The model under review builds one solid part; all positions refer to its coordinate system, in mm. A direction names the side the tool comes from. Round coordinates to 2 decimals unless told otherwise and drop trailing zeros. Order: outer loops, then holes, each group sorted by start corner. A loop starts at its lowest first (then second) coordinate and runs counter-clockwise, first axis right, second up. Notation, with made-up numbers: M 77.5,88 L 128.5,88 A23 cw 128.5,115 Z; hole C 43,7 d9. An arc over 180 degrees is marked long. Answer as a JSON object with one key per item and string values. Group by question number.
1. Add section A-A on y = -9. State the section outline as (x, z) points.
2. Mouldability with a two-part tool opening along Y and no side actions: class faces 4 (the face through (-44.44, -49.53, 67.02)), 5 (the face through (3, -17, 29.674)), 6 (the face through (2, 12.931, 37)), 7 (the face through (-25, -52.069, 37)) as released by +Y, released by -Y, zero draft, split by the parting line, or undercut.
3. Machinability: for faces 1 (the face through (3, -17, 43.524)), 2 (the face through (2, -34, 75)), 3 (the face through (-27, -47.069, 37)), which of the approach directions +Z, -Z, +X, -X, +Y, -Y give a long, thin tool a straight path to every point of the face, cutting with its end or side? Answer none if there is none.
4. Clearance check with flat-ended pins moving along their axes: P1, Ø3, axis at x = -17, z = 61, coming from the +Y side; P2, Ø2.5, axis at y = -2.46, z = 36.6, coming from the -X side. State where each tip first meets the part, or that it passes through.
5. To check wall thickness, follow probe 1 along Y at (x, z) = (-36.5, 72.5); probe 2 along X at (y, z) = (-33.5, 5). State the ranges of each line that lie inside material, in increasing order. Write a range as [from, to].
6. Add section C-C on z = 67. State the section outline as (x, y) points.
7. Add section B-B on z = 31. State the section outline as (x, y) points.
8. Add section D-D on x = -19.5. State the section outline as (y, z) points, and give its area (3 significant figures).
Autodesk Inventor part; units mm, degrees
ref_plane "YZ Plane" through (0, 0, 0) normal (1, 0, 0) x (0, 1, 0)
ref_plane "XZ Plane" through (0, 0, 0) normal (0, 1, 0) x (-1, 0, 0)
ref_plane "XY Plane" through (0, 0, 0) normal (0, 0, 1) x (1, 0, 0)
sketch "Sketch1" plane through (0, 0, 0) normal (0, 0, 1) x (1, 0, 0)
  point P0 (0, 0)
sketch "Sketch2" plane through (0, 0, 0) normal (0, 0, 1) x (1, 0, 0)
  line L0 (0, 12.9308) -> (5, 12.9308)
  line L1 (5, 12.9308) -> (5, -47.0692)
  line L2 (0, -47.0692) -> (0, 12.9308)
  line L3 (0, -47.0692) -> (-55, -47.0692)
  line L4 (-55, -47.0692) -> (-55, -52.0692)
  line L5 (-55, -52.0692) -> (5, -52.0692)
  line L6 (5, -52.0692) -> (5, -47.0692)
  point P0 (0, 0)
extrude "Extrusion1" add sketch "Sketch2" along normal blind 75
sketch "Sketch3" plane through (-55, -47.0692, 0) normal (0, 1, 0) x (1, 0, 0)
  circle A0 centre (8.2492, -7.6821) radius 2.5
  circle A1 centre (8.2492, -66.0616) radius 2.5
  point P0 (55, 0)
  dimension "d6" = 5
  dimension "d7" = 5
extrude "Extrusion2" cut sketch "Sketch3" against normal blind 75
sketch "Sketch4" plane through (5, -52.0692, 0) normal (1, 0, 0) x (0, 0, -1)
  line L0 (-43.5238, 46.3128) -> (-29.6738, 46.3128)
  line L1 (-29.6738, 46.3128) -> (-29.6738, 23.4735)
  line L2 (-29.6738, 23.4735) -> (-43.5238, 23.4735)
  line L3 (-43.5238, 23.4735) -> (-43.5238, 46.3128)
  point P0 (0, 52.0692)
extrude "Extrusion3" cut sketch "Sketch4" against normal blind 75
sketch "Sketch5" plane through (5, -52.0692, 0) normal (1, 0, 0) x (0, 0, -1)
  line L0 (-43.5238, 46.3128) -> (-43.5238, 23.4735)
  line L1 (-43.5238, 46.3128) -> (-29.6738, 46.3128)
  line L2 (-43.5238, 46.3128) -> (-29.6738, 46.3128)
  line L3 (-43.5238, 46.3128) -> (-36.5988, 46.3128)
  circle A0 centre (-36.5988, 49.6128) radius 1
  circle A1 centre (-36.5988, 20.1735) radius 1
  point P0 (0, 52.0692)
extrude "Extrusion4" cut sketch "Sketch5" against normal blind 75
Recorded:
{
 "1": {"outline": "M 0,0 L 5,0 L 5,29.67 L 0,29.67 Z; M 0,43.52 L 5,43.52 L 5,75 L 0,75 Z"},
 "2": {"face 4": "zero draft", "face 5": "undercut", "face 6": "released by +Y", "face 7": "released by -Y"},
 "3": {"face 1": "+X, -X", "face 2": "+Z, +X, -X, +Y, -Y", "face 3": "+Z, -Z, -X, +Y"},
 "4": {"P1": "stops at y = -47.07", "P2": "stops at x = 0"},
 "5": {"probe 1": "y = [-52.07, -47.07]", "probe 2": "x = [0, 5]"},
 "6": {"outline": "M -55,-52.07 L -49.07,-52.07 L -49.07,-47.07 L -55,-47.07 Z; M -44.43,-52.07 L 5,-52.07 L 5,12.93 L 0,12.93 L 0,-47.07 L -44.43,-47.07 Z"},
 "7": {"outline": "M -55,-52.07 L 5,-52.07 L 5,-28.6 L 0,-28.6 L 0,-47.07 L -55,-47.07 Z; M 0,-5.76 L 5,-5.76 L 5,12.93 L 0,12.93 Z"},
 "8": {"outline": "M -52.07,0 L -47.07,0 L -47.07,75 L -52.07,75 Z", "area": "375 mm²"}
}
